```python
from build123d import *

# Parameters (mm, degrees)
ESTRUSIONE_ESTRUSIONE1_DEPTH = 25
SCHIZZO2_R                   = 7.5
TAGLIO_ESTRUSIONE1_DEPTH     = 47.435439053
SCHIZZO3_W                   = 7
SCHIZZO3_H                   = 1.4
TAGLIO_ESTRUSIONE2_DEPTH     = 47.435439053
RACCORDO2_R                  = 1


with BuildPart() as part:
    # Schizzo1 → Estrusione-Estrusione1 (new body)
    with BuildSketch(Plane.XY):
        with BuildLine():
            Line((-4, -14.085786438), (-4, -16.5))
            ThreePointArc((-4, -16.5), (-4.292893219, -17.207106781), (-5, -17.5))
            Line((-5, -17.5), (-17.5, -17.5))
            Line((-17.5, -17.5), (-17.5, 17.5))
            Line((-17.5, 17.5), (17.5, 17.5))
            Line((17.5, 17.5), (17.5, -17.5))
            Line((17.5, -17.5), (5, -17.5))
            ThreePointArc((5, -17.5), (4.292893219, -17.207106781), (4, -16.5))
            Line((4, -16.5), (4, -14.085786438))
            ThreePointArc((4, -14.085786438), (0, -10.085786438), (-4, -14.085786438))
        make_face()
    extrude(amount=ESTRUSIONE_ESTRUSIONE1_DEPTH)

    # Schizzo2 → Taglio-Estrusione1 (cut, through all)
    with BuildSketch(Plane(origin=(17.5, 0, 0), x_dir=(0, 0, -1), z_dir=(1, 0, 0))):
        with Locations(Location((-12.5, 6, 0), (0, 0, 90))):
            Circle(SCHIZZO2_R)
    extrude(amount=-TAGLIO_ESTRUSIONE1_DEPTH, mode=Mode.SUBTRACT)

    # Schizzo3 → Taglio-Estrusione2 (cut, through all)
    with BuildSketch(Plane(origin=(17.5, 0, 0), x_dir=(0, 0, -1), z_dir=(1, 0, 0))):
        with Locations((-12.5, -6.385786438)):
            Rectangle(SCHIZZO3_W, SCHIZZO3_H)
    extrude(amount=-TAGLIO_ESTRUSIONE2_DEPTH, mode=Mode.SUBTRACT)

    # Raccordo2
    raccordo2_edges = [part.edges().sort_by_distance(p)[0] for p in [
        (-4.292893219, -17.207106781, 25),
        (11.25, -17.5, 0),
        (4.292893219, -17.207106781, 0),
        (4, -15.292893219, 0),
        (0, -10.085786438, 0),
        (-4, -15.292893219, 0),
        (-4.292893219, -17.207106781, 0),
        (-11.25, -17.5, 0),
        (-17.5, 0, 0),
        (-4, -15.292893219, 25),
        (0, -10.085786438, 25),
        (-17.5, 17.5, 12.5),
        (17.5, 17.5, 12.5),
        (17.5, -17.5, 12.5),
        (-17.5, -17.5, 12.5),
        (4, -15.292893219, 25),
        (4.292893219, -17.207106781, 25),
        (11.25, -17.5, 25),
        (17.5, 0, 25),
        (0, 17.5, 25),
        (-17.5, 0, 25),
        (-11.25, -17.5, 25),
        (0, 17.5, 0),
        (17.5, 0, 0),
    ]]
    fillet(raccordo2_edges, radius=RACCORDO2_R)


solid = part.part
```
Work out the finished part from the listing and answer in its coordinate system (mm). A direction names the side the tool comes from. Give positions to 0.01 mm unless a question says otherwise; leave off trailing zeros. Loops run counter-clockwise (first coordinate to the right, second up) from the corner with the lowest first, then second, coordinate; pieces in that order, holes last. Notation, with made-up numbers: (81, 34.5) -> (86, 34.5) arc R24 cw to (86, 50.5) -> close; hole circle Ø1 at (15.5, -25.75). An arc over 180 degrees is marked (long way). Put each result on its own line as item: value. Start each with the question number.
Item 1: Find the intervals of material crossed by L1, parallel to Z at x = 9.5, y = -6.5; L2, parallel to Z at x = -7, y = 6; L3, parallel to Y at x = 10, z = 12.25, in increasing order. Write a range as [from, to].
Item 2: Which of the six approach directions +Z, -Z, +X, -X, +Y, -Y give full straight-line access (tool end or side, diameter ignored) to faces 5 (the face through (4.301, -15.276, 0.285)), 6 (the face through (4.301, -17.215, 12.339)), 7 (the face through (0, -7.086, 13))?
Item 3: The part is cut by section A-A (y = 0). Give the vertices of the cut face in (x, z), then the cut area to 3 significant figures.
Item 4: The part is cut by section B-B (x = 0). Give the vertices of the cut face in (y, z), then the cut area to 3 significant figures.
Item 5: The mould has two halves that part along X. Classify faces 1 (the face through (17.215, -17.199, 12.661)), 2 (the face through (-4.285, -15.31, 24.699)), 3 (the face through (0.231, 17.199, 0.285)), 4 (the face through (-17.215, 17.199, 12.661)): released by +X, released by -X, zero draft, split by the parting line, or undercut.
Item 6: The part is cut by section C-C (z = 13.5). Give the vertices of the cut face in (x, y).
Item 7: The part is cut by section D-D (y = -15). Give the vertices of the cut face in (x, z).
Answers below:
1. L1: [0, 9], [16, 25]
1. L2: [0, 5], [20, 25]
1. L3: [-17.5, -7.09], [-5.69, -1.5], [13.5, 17.5]
2. face 5: -Z, -Y
2. face 6: +Z, -Z, -Y
2. face 7: +X, -X
3. outline: (-17.5, 1) arc R1 ccw to (-16.5, 0) -> (16.5, 0) arc R1 ccw to (17.5, 1) -> (17.5, 8) -> (-17.5, 8) -> close; (-17.5, 17) -> (17.5, 17) -> (17.5, 24) arc R1 ccw to (16.5, 25) -> (-16.5, 25) arc R1 ccw to (-17.5, 24) -> close
3. area: 559 mm2
4. outline: (-10.09, 1) arc R1 ccw to (-9.09, 0) -> (16.5, 0) arc R1 ccw to (17.5, 1) -> (17.5, 24) arc R1 ccw to (16.5, 25) -> (-9.09, 25) arc R1 ccw to (-10.09, 24) -> close; hole (-7.09, 9) -> (-5.69, 9) -> (-5.69, 16) -> (-7.09, 16) -> close; hole circle Ø15 at (6, 12.5)
4. area: 502 mm2
5. face 1: released by +X
5. face 2: undercut
5. face 3: zero draft
5. face 4: released by -X
6. outline: (-17.5, -16.5) arc R1 ccw to (-16.5, -17.5) -> (-5, -17.5) arc R1 ccw to (-4, -16.5) -> (-4, -14.09) arc R4 cw to (4, -14.09) -> (4, -16.5) arc R1 ccw to (5, -17.5) -> (16.5, -17.5) arc R1 ccw to (17.5, -16.5) -> (17.5, -7.09) -> (-17.5, -7.09) -> close; (-17.5, -5.69) -> (17.5, -5.69) -> (17.5, -1.43) -> (-17.5, -1.43) -> close; (-17.5, 13.43) -> (17.5, 13.43) -> (17.5, 16.5) arc R1 ccw to (16.5, 17.5) -> (-16.5, 17.5) arc R1 ccw to (-17.5, 16.5) -> close
7. outline: (-17.5, 1) arc R1 ccw to (-16.5, 0) -> (-5, 0) arc R1 ccw to (-4, 1) -> (-4, 24) arc R1 ccw to (-5, 25) -> (-16.5, 25) arc R1 ccw to (-17.5, 24) -> close; (4, 1) arc R1 ccw to (5, 0) -> (16.5, 0) arc R1 ccw to (17.5, 1) -> (17.5, 24) arc R1 ccw to (16.5, 25) -> (5, 25) arc R1 ccw to (4, 24) -> close
